from build123d import *

# Parameters (mm, degrees)
F0_R     = 2.85
F1_DEPTH = 3
F2_SIZE2 = 0.6
F2_SIZE  = 0.4
F3_R     = 1.45
F4_DEPTH = 2
F5_R     = 1.95
F5_R_2   = 1.45
F6_DEPTH = 0.5
F7_SIZE  = 0.2
F8_R     = 4.45
F8_R_2   = 2.45
F9_DEPTH = 0.2


with BuildPart() as f1:
    # F0 (on Right) → F1 (new body)
    with BuildSketch(Plane.YZ):
        Circle(F0_R)
    extrude(amount=F1_DEPTH)

    # F2
    f2_edges = [f1.edges().sort_by_distance(p)[0] for p in [
        (3, -2.85, 0),
    ]]
    f2_side = f1.faces().sort_by_distance((3, 0, 0))[0]
    chamfer(f2_edges, length=F2_SIZE, length2=F2_SIZE2, reference=f2_side)

    # F3 (on face) → F4 (join)
    with BuildSketch(Plane(origin=(0, 0, 0), x_dir=(0, -1, 0), z_dir=(-1, 0, 0))):
        Circle(F3_R)
    extrude(amount=F4_DEPTH)

    # F5 (on face) → F6 (cut)
    with BuildSketch(Plane(origin=(0, 0, 0), x_dir=(0, -1, 0), z_dir=(-1, 0, 0))):
        Circle(F5_R)
        Circle(F5_R_2, mode=Mode.SUBTRACT)
    extrude(amount=-F6_DEPTH, mode=Mode.SUBTRACT)

    # F7
    f7_edges = [f1.edges().sort_by_distance(p)[0] for p in [
        (0.5, 1.95, 0),
    ]]
    chamfer(f7_edges, length=F7_SIZE)

    # F8 (on face) → F9 (join)
    with BuildSketch(Plane.YZ.offset(3)):
        Circle(F8_R)
        Circle(F8_R_2, mode=Mode.SUBTRACT)
    extrude(amount=-F9_DEPTH)


solid = f1.part
The listing builds one solid part. Answer for the finished solid, in the listing's coordinates (mm). A direction names the side the tool comes from. Give positions to 0.01 mm unless a question says otherwise; leave off trailing zeros. Write each loop counter-clockwise with the first axis right and the second up, starting at its lowest first coordinate (ties: lowest second). Pieces come first, ordered by that corner, then holes. Notation, with made-up numbers: (88, -16) -> (107, -16) arc R29 cw to (107, 6) -> close; hole circle Ø7 at (14, 64). An arc over 180 degrees is marked (long way). Use a Markdown table: item, result.
(1) Determine the mould class of faces 3 (the flat face through (2.8, 2, -2)), 4 (the cylindrical face through (1.183, -2.262, -1.734)), 5 (the cylindrical face through (-0.77, 1.45, 0.06)) for opening direction Z: released by +Z, released by -Z, zero draft, split by the parting line, or undercut.
Return value:
| item | result |
|---|---|
| face 3 | zero draft |
| face 4 | split by the parting line |
| face 5 | undercut |
(2) Find the intervals of material crossed by probe 1 along Z at (x, y) = (0.1, 0); probe 2 along Y at (x, z) = (0.05, -0.5); probe 3 along X at (y, z) = (0.5, 1.5), in increasing order. Write a range as from..to.
Return value:
| item | result |
|---|---|
| probe 1 | -2.85..-1.95, -1.45..1.45, 1.95..2.85 |
| probe 2 | -2.81..-1.88, -1.36..1.36, 1.88..2.81 |
| probe 3 | 0.5..3 |
(3) Section D-D, the plane x = 1.1 is taken. Determine the outline of the cut face in (y, z), then the cut area to 3 significant figures.
Return value:
| item | result |
|---|---|
| outline | circle Ø5.7 at (0, 0) |
| area | 25.5 mm2 |
(4) Section A-A, the plane y = 0 is taken. Determine the outline of the cut face in (x, z).
Return value:
| item | result |
|---|---|
| outline | (-2, -1.45) -> (0.5, -1.45) -> (0.5, -1.75) -> (0.3, -1.95) -> (0, -1.95) -> (0, -2.85) -> (2.4, -2.85) -> (2.8, -2.58) -> (2.8, -4.45) -> (3, -4.45) -> (3, 4.45) -> (2.8, 4.45) -> (2.8, 2.58) -> (2.4, 2.85) -> (0, 2.85) -> (0, 1.95) -> (0.3, 1.95) -> (0.5, 1.75) -> (0.5, 1.45) -> (-2, 1.45) -> close |
(5) For faces 1 (the flat face through (0, 1, -2)), 2 (the flat face through (-2, 0, 0)), determine the directions among +Z, -Z, +X, -X, +Y, -Y from which every point of the face is accessible in a straight line to the end or side of a thin tool.
Return value:
| item | result |
|---|---|
| face 1 | -X |
| face 2 | +Z, -Z, -X, +Y, -Y |
(6) Flat-ended cylindrical pins translate along their axes: P1, Ø1.5, axis at x = 0.5, z = -0.5, coming from the -Y side; P2, Ø1.5, axis at y = -2, z = -1.5, coming from the -X side; P3, Ø1.5, axis at x = 1, y = -2, coming from the +Z side. Find the tip coordinate at first contact, or state that the pin passes through.
Return value:
| item | result |
|---|---|
| P1 | y = -2.85 |
| P2 | x = 0 |
| P3 | z = 2.56 |
(7) Section B-B, the plane x = -0.9 is taken. Determine the outline of the cut face in (y, z).
Return value:
| item | result |
|---|---|
| outline | circle Ø2.9 at (0, 0) |
